from build123d import *

# Parameters (mm, degrees)
F0_W     = 404
F0_H     = 317
F1_DEPTH = 8
F2_W     = 8
F2_H     = 19
F2_H_2   = 23
F2_W_2   = 24
F2_H_3   = 24
F3_DEPTH = 8
F5_DEPTH = 8.001


with BuildPart() as f1:
    # F0 (on Top) → F1 (new body)
    with BuildSketch(Plane.XY):
        Rectangle(F0_W, F0_H)
    extrude(amount=F1_DEPTH)

    # F2 (on face) → F3 (cut)
    with BuildSketch(Plane.XY.offset(8)):
        with Locations((-198, -120)):
            Rectangle(F2_W, F2_H)
        Polygon((-202, 35.5), (-202, -35.5), (-197, -35.5), (-197, -9.5), (-192, -9.5), (-192, 9.5), (-197, 9.5), (-197, 35.5), align=None)
        with Locations((-198, 107)):
            Rectangle(F2_W, F2_H_2)
        with Locations((-190, 138.5)):
            Rectangle(F2_W_2, F2_H_3)
        Polygon((192, -9.5), (197, -9.5), (197, -35.5), (202, -35.5), (202, 35.5), (197, 35.5), (197, 9.5), (192, 9.5), align=None)
        with Locations((198, -120)):
            Rectangle(F2_W, F2_H)
        with Locations((198, 107)):
            Rectangle(F2_W, F2_H_2)
        with Locations((190, 138.5)):
            Rectangle(F2_W_2, F2_H_3)
    extrude(amount=-F3_DEPTH, mode=Mode.SUBTRACT)

    # F4 (on face) → F5 (cut, through all)
    with BuildSketch(Plane.XY.offset(8)):
        with BuildLine():
            Line((-175, 56.5), (-175, -46.5))
            Line((-175, -46.5), (-140, -46.5))
            Line((-140, -46.5), (-140, 38.5))
            Line((-140, 38.5), (-122, 56.5))
            Line((-122, 56.5), (-53.216133, 56.5))
            Line((-53.216133, 56.5), (-53.216133, 44.5))
            ThreePointArc((-53.216133, 44.5), (-48.529842, 33.186292), (-37.216133, 28.5))
            Line((-37.216133, 28.5), (37.216133, 28.5))
            ThreePointArc((37.216133, 28.5), (48.529842, 33.186292), (53.216133, 44.5))
            Line((53.216133, 44.5), (53.216133, 56.5))
            Line((53.216133, 56.5), (122, 56.5))
            Line((122, 56.5), (140, 38.5))
            Line((140, 38.5), (140, -46.5))
            Line((140, -46.5), (175, -46.5))
            Line((175, -46.5), (175, 56.5))
            Line((175, 56.5), (129, 102.5))
            Line((129, 102.5), (-129, 102.5))
            Line((-129, 102.5), (-175, 56.5))
        make_face()
    extrude(amount=-F5_DEPTH, mode=Mode.SUBTRACT)


solid = f1.part
Source: CAD feature listing. Evaluate the final solid. Frame: model axes, mm. A direction names the side the tool comes from. Coordinates: 2 decimals unless noted, no trailing zeros. Loops run counter-clockwise (first coordinate to the right, second up) from the corner with the lowest first, then second, coordinate; pieces in that order, holes last. Notation, with made-up numbers: (57.5, -18) - (66.5, -18) arc R33 ccw to (66.5, 10) - close; hole circle Ø7 at (-37, 7.25). An arc over 180 degrees is marked (long way). Return JSON: item names as keys, results as strings.
Q1. Section C-C, the plane y = -30. Return loops of the section in (x, z), plus the area to 3 significant figures.
Results:
{"outline": "(-197, 0) - (-175, 0) - (-175, 8) - (-197, 8) - close; (-140, 0) - (140, 0) - (140, 8) - (-140, 8) - close; (175, 0) - (197, 0) - (197, 8) - (175, 8) - close", "area": "2,590 mm2"}
Q2. Mould query, pull axis Y, two halves, no side actions, for faces 1 (the flat face through (-1, 28.5, 4)), 2 (the flat face through (-3, 158.5, 4)), 3 (the flat face through (-202, 65, 4)), 4 (the flat face through (-175, 6, 4)). Classes: released by +Y, released by -Y, zero draft, split by the parting line, or undercut.
Results:
{"face 1": "undercut", "face 2": "released by +Y", "face 3": "zero draft", "face 4": "undercut"}
Q3. Section A-A, the plane y = 71. Return loops of the section in (x, z).
Results:
{"outline": "(-202, 0) - (-160.5, 0) - (-160.5, 8) - (-202, 8) - close; (160.5, 0) - (202, 0) - (202, 8) - (160.5, 8) - close"}
Q4. Section B-B, the plane x = -169. Return loops of the section in (y, z).
Results:
{"outline": "(-158.5, 0) - (-46.5, 0) - (-46.5, 8) - (-158.5, 8) - close; (62.5, 0) - (158.5, 0) - (158.5, 8) - (62.5, 8) - close"}
Q5. Access query for faces 5 (the flat face through (-202, 122, 4)), 6 (the flat face through (87, 56.5, 4)), 7 (the flat face through (202, -144, 4)), 8 (the flat face through (-198, 118.5, 4)), 9 (the flat face through (190, 126.5, 4)). Directions: +Z, -Z, +X, -X, +Y, -Y. A direction counts if a zero-diameter tool reaches every point of the face in a straight line with its end or side. Return the directions, or none.
Results:
{"face 5": "+Z, -Z, -X, +Y, -Y", "face 6": "+Z, -Z", "face 7": "+Z, -Z, +X, +Y, -Y", "face 8": "+Z, -Z, -X", "face 9": "+Z, -Z, +X"}
Q6. Contact query for a flat-ended pin moving along its axis: P1, Ø4, axis at y = -121.5, z = 3, coming from the -X side. Output: stop coordinate, or through.
Results:
{"P1": "x = -194"}
Q7. Material intervals for line 1 along Y through (x, z) = (30, 2); line 2 along Y through (x, z) = (-105.5, 1); line 3 along X through (y, z) = (130.5, 5.25), sorted ascending.
Results:
{"line 1": "-158.5 to 28.5, 102.5 to 158.5", "line 2": "-158.5 to 56.5, 102.5 to 158.5", "line 3": "-178 to 178"}
